from build123d import *

# Parameters (mm, degrees)
F1_DEPTH = 50
F2_R     = 15
F3_DEPTH = 51
F4_R     = 10
F5_DEPTH = 51


with BuildPart() as f1:
    # F0 (on Front) → F1 (new body)
    with BuildSketch(Plane.XZ):
        with BuildLine():
            Line((-57.174233, 36.999495), (-87.174233, 36.999495))
            Line((-87.174233, 36.999495), (-87.174233, 11.999495))
            Line((-87.174233, 11.999495), (52.825767, 11.999495))
            Line((52.825767, 11.999495), (52.825767, 36.999495))
            Line((52.825767, 36.999495), (22.825767, 36.999495))
            Line((22.825767, 36.999495), (22.825767, 76.999495))
            ThreePointArc((22.825767, 76.999495), (-17.174233, 116.999495), (-57.174233, 76.999495))
            Line((-57.174233, 76.999495), (-57.174233, 36.999495))
        make_face()
    extrude(amount=F1_DEPTH)

    # F2 (on face) → F3 (cut)
    with BuildSketch(Plane.XZ.offset(50)):
        with Locations((-17.19176, 76.999495)):
            Circle(F2_R)
    extrude(amount=-F3_DEPTH, mode=Mode.SUBTRACT)

    # F4 (on face) → F5 (cut)
    with BuildSketch(Plane.XY.offset(36.999495)):
        with Locations((-72.174233, -25)):
            Circle(F4_R)
        with Locations((37.825767, -25)):
            Circle(F4_R)
    extrude(amount=-F5_DEPTH, mode=Mode.SUBTRACT)


solid = f1.part
Verification items for the finished model (mm, model axes). A direction names the side the tool comes from. Give positions to 0.01 mm unless a question says otherwise; leave off trailing zeros. Write each loop counter-clockwise with the first axis right and the second up, starting at its lowest first coordinate (ties: lowest second). Pieces come first, ordered by that corner, then holes. Notation, with made-up numbers: M 2,23.5 L 44,23.5 A11 ccw 44,42.5 Z; hole C 51,13 d3. An arc over 180 degrees is marked long. Use CSV: the item, a comma, the result in double quotes.
1) Release check for a two-part mould opening along Y. For faces 1 (the face through (-18, 0, 54)), 2 (the face through (-62.636, -21.996, 24.674)), 3 (the face through (-62, -25, 36.999)) record: released by +Y, released by -Y, zero draft, split by the parting line, or undercut.
Final values:
face 1,"released by +Y"
face 2,"undercut"
face 3,"zero draft"
2) Access from +Z, -Z, +X, -X, +Y, -Y to the whole of each face (thin tool, end or side, straight path). Record for faces 4 (the face through (22.826, -25, 57)), 5 (the face through (-87.174, -25, 25)), 6 (the face through (-57.174, -25, 57)).
Final values:
face 4,"+Z, +X, +Y, -Y"
face 5,"+Z, -Z, -X, +Y, -Y"
face 6,"+Z, -X, +Y, -Y"
3) Go/stop test with flat-tipped pins: pin 1 Ø2 at (y, z) = (-23.5, 61.5) entering from +X; pin 2 Ø15 at (x, y) = (34, -21) entering from +Z; pin 3 Ø1.5 at (y, z) = (-14, 53.5) entering from -X. Record where each tip stops, or that it passes through.
Final values:
pin 1,"x = 22.83"
pin 2,"z = 37"
pin 3,"x = -57.17"
4) Cross-section at D-D (z = 85.5). Enter the section's corners in (x, y).
Final values:
outline,"M -56.26,-50 L -29.55,-50 L -29.55,0 L -56.26,0 Z; M -4.83,-50 L 21.91,-50 L 21.91,0 L -4.83,0 Z"
5) Cross-section at B-B (x = -10). Enter the section's corners in (y, z), plus the area to 3 significant figures.
Final values:
outline,"M -50,12 L 0,12 L 0,63.84 L -50,63.84 Z; M -50,90.16 L 0,90.16 L 0,116.35 L -50,116.35 Z"
area,"3,900 mm²"
6) Cross-section at C-C (y = -11). Enter the section's corners in (x, z).
Final values:
outline,"M -87.17,12 L 52.83,12 L 52.83,37 L 22.83,37 L 22.83,77 A40 ccw -57.17,77 L -57.17,37 L -87.17,37 Z; hole C -17.19,77 d30"
7) Material ranges on line 1 along Y through (x, z) = (37, 36.5); line 2 along X through (y, z) = (-19.5, 32); line 3 along Z through (x, y) = (-11.5, -37.5), recorded low to high.
Final values:
line 1,"-50 to -34.97, -15.03 to 0"
line 2,"-87.17 to -80.53, -63.82 to 29.47, 46.18 to 52.83"
line 3,"12 to 63.12, 90.88 to 116.59"
8) Cross-section at A-A (y = -25). Enter the section's corners in (x, z).
Final values:
outline,"M -87.17,12 L -82.17,12 L -82.17,37 L -87.17,37 Z; M -62.17,12 L 27.83,12 L 27.83,37 L 22.83,37 L 22.83,77 A40 ccw -57.17,77 L -57.17,37 L -62.17,37 Z; M 47.83,12 L 52.83,12 L 52.83,37 L 47.83,37 Z; hole C -17.19,77 d30"
